Geometry: final body of the model. Coordinates: model frame, mm. Coordinates: 2 decimals unless noted, no trailing zeros. Order: outer loops, then holes, each group sorted by start corner. A loop starts at its lowest first (then second) coordinate and runs counter-clockwise, first axis right, second up. Notation, with made-up numbers: (4.5, -39) -> (58.5, -39) arc R11 cw to (58.5, -30) -> close; hole circle Ø10 at (35.5, 34). An arc over 180 degrees is marked (long way). Answer in a Markdown table with one row per item. Add a question column.
1) Section query A-A on y = 0. Return the cut outline in (x, z), then the cut area to 3 significant figures.
2) Contact query for flat-ended pins moving along their axis: P1, Ø2, axis at x = 162.5, y = -14.5, coming from the +Z side; P2, Ø2, axis at x = 30, y = -8, coming from the -Z side; P3, Ø1.6, axis at x = 4, y = -13.5, coming from the -Z side. Output: stop coordinate, or through.
3) Ray query, line 1 (Z direction, x = 100, y = 0); line 2 (Y direction, x = 146.5, z = 2.5). Return the intervals inside material, ascending. Write a range as from..to.
4) Section query C-C on z = -9.5. Return the cut outline in (x, y).
5) Pull-direction query (Z, two-part tool) for faces 1 (the face through (81.345, 13.856, 5.745)), 2 (the face through (165, 6, -12)), 3 (the face through (81.3, 12.4, -3.9)); classes: +Z half, -Z half, draft (parallel to the pull), parting line (faces both ways), or undercut.
6) Section query B-B on x = 91. Return the cut outline in (y, z), then the cut area to 3 significant figures.
Autodesk Inventor part; units mm, degrees
ref_plane "Work Plane1" through (82.5, 0, 0) normal (-1, 0, 0) x (0, 0, 1)
ref_plane "Work Plane2" through (0, -15, 0) normal (0, 1, 0) x (-1, 0, 0)
ref_plane "YZ Plane" through (0, 0, 0) normal (1, 0, 0) x (0, 1, 0)
sketch "Sketch1" plane through (0, 0, 0) normal (1, 0, 0) x (0, 1, 0)
  circle A0 centre (0, 0) radius 15
  circle A1 centre (0, 0) radius 13
  dimension "d0" = 30
  dimension "d1" = 26
extrude "Extrusion1" add sketch "Sketch1" along normal blind 165
sketch "Sketch2" plane through (0, 0, 0) normal (0, 1, 0) x (-1, 0, 0)
  line L0 (0, 0) -> (-165, 0) construction
  line L1 (-165, 15) -> (-165, -15) construction
  line L2 (-11, 2) -> (0, 2)
  line L3 (0, 2) -> (0, -2)
  line L4 (0, -2) -> (-11, -2)
  line L5 (-11, -2) -> (-11, 2)
  line L6 (-11, 2) -> (0, -2)
  line L7 (0, 2) -> (-11, -2)
  line L8 (0, -15) -> (0, 15)
  line L9 (0, 15) -> (0, -15)
  line L10 (0, -15) -> (-165, -15)
  point P0 (-5.5, 0)
  dimension "d4" = 4
  dimension "d5" = 11
extrude "Extrusion2" cut sketch "Sketch2" against normal through all
fillet "Fillet1" radius 2 2 edges at (11, -13.8557, 2) (11, -13.8557, -2)
ref_plane "Work Plane1" through (82.5, 0, 0) normal (-1, 0, 0) x (0, 0, 1)
mirror "Mirror1" about plane through (82.5, 0, 0) normal (-1, 0, 0) of "Extrusion2", "Fillet1"
ref_plane "Work Plane2" through (0, -15, 0) normal (0, 1, 0) x (-1, 0, 0)
properties part number "Laser_tube" material "Polycarbonate, Clear"
Result:
| question | item | result |
|---|---|---|
| 1 | outline | (0, -15) -> (165, -15) -> (165, -13) -> (0, -13) -> close; (0, 13) -> (165, 13) -> (165, 15) -> (0, 15) -> close |
| 1 | area | 660 mm2 |
| 2 | P1 | z = 6.54 |
| 2 | P2 | z = -13.27 |
| 2 | P3 | z = -7.98 |
| 3 | line 1 | -15..-13, 13..15 |
| 3 | line 2 | -14.79..-12.76, 12.76..14.79 |
| 4 | outline | (0, -11.61) -> (165, -11.61) -> (165, -8.87) -> (0, -8.87) -> close; (0, 8.87) -> (165, 8.87) -> (165, 11.61) -> (0, 11.61) -> close |
| 5 | face 1 | parting line |
| 5 | face 2 | draft |
| 5 | face 3 | undercut |
| 6 | outline | circle Ø30 at (0, 0); hole circle Ø26 at (0, 0) |
| 6 | area | 176 mm2 |
